Source: CAD feature listing. Evaluate the final solid. Frame: model axes, mm. Round coordinates to 2 decimals unless told otherwise and drop trailing zeros. Order: outer loops, then holes, each group sorted by start corner. A loop starts at its lowest first (then second) coordinate and runs counter-clockwise, first axis right, second up. Notation, with made-up numbers: M 30.5,8 L 73.5,8 A17 cw 73.5,15 Z; hole C 15,69 d11. An arc over 180 degrees is marked long. Answer as CSV lines item,"result". Start each with the question number.
Item 1: Section query A-A on x = -17. Return the cut outline in (y, z).
Item 2: Line query: line 1 (Z direction, x = 13, y = -0.8); line 2 (X direction, y = -0.6, z = -1.5) (3 decimals). Output: solid intervals per line, ascending. Write a range as [from, to].
Item 3: Section query B-B on z = 2. Return the cut outline in (x, y) (3 decimals).
Item 4: First-contact query: P1, Ø0.8, axis at y = 0.5, z = -42, coming from the -X side; P2, Ø1, axis at y = 0, z = 5, coming from the +X side (3 decimals); P3, Ø0.9, axis at y = 0, z = 47.5, coming from the -X side (3 decimals). Flat tips, straight axial feed; report the tip coordinate or a pass-through.
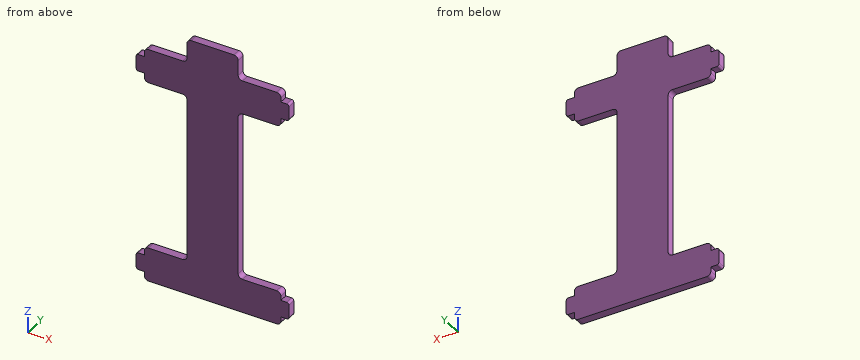
from build123d import *

# Parameters (mm, degrees)
BOSS_EXTRUDE1_DEPTH = 1.5
FILLET1_R           = 1.5875
SKETCH2_W           = 3
SKETCH2_H           = 6.35
BOSS_EXTRUDE2_DEPTH = 3
FILLET2_R           = 0.79375


with BuildPart() as part:
    # Sketch1 → Boss-Extrude1 (new, symmetric)
    with BuildSketch(Plane(origin=(0, 0, 0), x_dir=(1, 0, 0), z_dir=(0, 1, 0))):
        Polygon((25.4, 31.75), (9.525, 31.75), (9.525, -31.75), (25.4, -31.75), (25.4, -44.45), (9.525, -44.45), (9.525, -53.34), (-9.525, -53.34), (-9.525, -44.45), (-25.4, -44.45), (-25.4, -31.75), (-9.525, -31.75), (-9.525, 31.75), (-25.4, 31.75), (-25.4, 44.45), (25.4, 44.45), align=None)
    extrude(amount=BOSS_EXTRUDE1_DEPTH, both=True)

    # Fillet1
    fillet1_edges = [part.edges().sort_by_distance(p)[0] for p in [
        (25.4, 0, -44.45),
        (25.4, 0, -31.75),
        (9.525, 0, -31.75),
        (9.525, 0, 31.75),
        (25.4, 0, 31.75),
        (25.4, 0, 44.45),
        (9.525, 0, 44.45),
        (9.525, 0, 53.34),
        (-9.525, 0, 53.34),
        (-9.525, 0, 44.45),
        (-25.4, 0, 44.45),
        (-25.4, 0, 31.75),
        (-9.525, 0, 31.75),
        (-9.525, 0, -31.75),
        (-25.4, 0, -31.75),
        (-25.4, 0, -44.45),
    ]]
    fillet(fillet1_edges, radius=FILLET1_R)

    # Sketch2 → Boss-Extrude2 (add)
    with BuildSketch(Plane(origin=(0, 1.5, 0), x_dir=(1, 0, 0), z_dir=(0, 1, 0))):
        with Locations((-26.9, 38.1)):
            Rectangle(SKETCH2_W, SKETCH2_H)
        with Locations((26.9, 38.1)):
            Rectangle(SKETCH2_W, SKETCH2_H)
        with Locations((26.9, -38.1)):
            Rectangle(SKETCH2_W, SKETCH2_H)
        with Locations((-26.9, -38.1)):
            Rectangle(SKETCH2_W, SKETCH2_H)
    extrude(amount=-BOSS_EXTRUDE2_DEPTH)

    # Fillet2
    fillet2_edges = [part.edges().sort_by_distance(p)[0] for p in [
        (-28.4, 0, 41.275),
        (-28.4, 0, 34.925),
        (28.4, 0, 34.925),
        (28.4, 0, 41.275),
        (28.4, 0, -41.275),
        (28.4, 0, -34.925),
        (-28.4, 0, -34.925),
        (-28.4, 0, -41.275),
    ]]
    fillet(fillet2_edges, radius=FILLET2_R)


solid = part.part
Results:
1,outline,"M -1.5,-44.45 L 1.5,-44.45 L 1.5,-31.75 L -1.5,-31.75 Z; M -1.5,31.75 L 1.5,31.75 L 1.5,44.45 L -1.5,44.45 Z"
2,line 1,"[-44.45, -31.75], [31.75, 44.45]"
2,line 2,"[-9.525, 9.525]"
3,outline,"M -9.525,-1.5 L 9.525,-1.5 L 9.525,1.5 L -9.525,1.5 Z"
4,P1,"x = -25.4"
4,P2,"x = 9.525"
4,P3,"x = -9.525"
